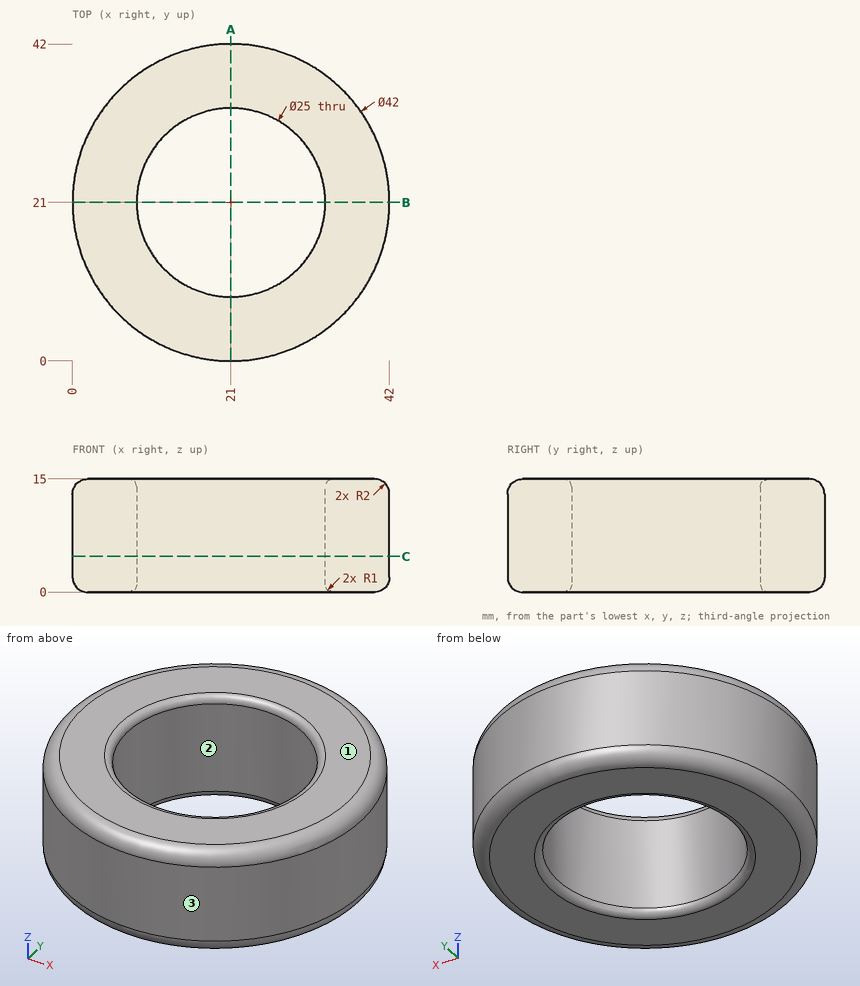
The drawing under review shows one solid part. Ordinate dimensions are in mm from its lowest x, y, z. Coordinates: 2 decimals unless noted, no trailing zeros. Loops run counter-clockwise (first coordinate to the right, second up) from the corner with the lowest first, then second, coordinate; pieces in that order, holes last.
Item 1: Clearance check with flat-ended pins moving along their axes: pin 1 (1.5 mm diameter, centred on y = 26.5, z = 2, fed in from +X); pin 2 (8 mm diameter, centred on x = 25, z = 3, fed in from +Y); pin 3 (2 mm diameter, centred on x = 32.5, z = 2, fed in from -Y); pin 4 (1.5 mm diameter, centred on x = 26, y = 30, fed in from +Z). State where each tip first meets the part, or that it passes through.
Completed:
pin 1: stops at x = 41.46
pin 2: stops at y = 42
pin 3: stops at y = 2.81
pin 4: passes through
Item 2: Add section A-A (x = 21). Write out the cut boundary in (y, z), and give its area (3 significant figures).
Completed:
outline: (0, 2) arc R2 ccw to (2, 0) - (7.5, 0) arc R1 ccw to (8.5, 1) - (8.5, 14) arc R1 ccw to (7.5, 15) - (2, 15) arc R2 ccw to (0, 13) - close; (33.5, 1) arc R1 ccw to (34.5, 0) - (40, 0) arc R2 ccw to (42, 2) - (42, 13) arc R2 ccw to (40, 15) - (34.5, 15) arc R1 ccw to (33.5, 14) - close
area: 251 mm2
Item 3: Add section C-C (z = 4.75). Write out the cut boundary in (x, y), and give its area (3 significant figures).
Completed:
outline: circle Ø42 at (21, 21); hole circle Ø25 at (21, 21)
area: 895 mm2
Item 4: Draft analysis for pull direction X (two halves, no side actions). For the marked faces 1, 2 and 3, state which applies: pulls with the +X half, pulls with the -X half, needs draft (parallel to the pull), parting line crosses it, or undercut.
Completed:
face 1: needs draft
face 2: undercut
face 3: parting line crosses it
Item 5: Wall thickness on L1, parallel to Y at x = 21, z = 10.25; L2, parallel to Y at x = 11, z = 1.5; L3, parallel to X at y = 32.5, z = 11: over which ranges is each line inside the solid? List them lowest first.
Completed:
L1: y = 0 to 8.5, 33.5 to 42
L2: y = 2.61 to 13.5, 28.5 to 39.39
L3: x = 3.43 to 16.1, 25.9 to 38.57
